Geometry check sheet. Reference: drawing and pictorial views, mm from the part's lowest x, y, z. A direction names the side the tool comes from. Coordinates: 2 decimals unless noted, no trailing zeros. Write each loop counter-clockwise with the first axis right and the second up, starting at its lowest first coordinate (ties: lowest second). Pieces come first, ordered by that corner, then holes. Notation, with made-up numbers: (-11.5, 88.25) -> (45.5, 88.25) arc R13 ccw to (45.5, 97.25) -> close; hole circle Ø7 at (78, -13.75). An arc over 180 degrees is marked (long way). Use a Markdown table: item, result.
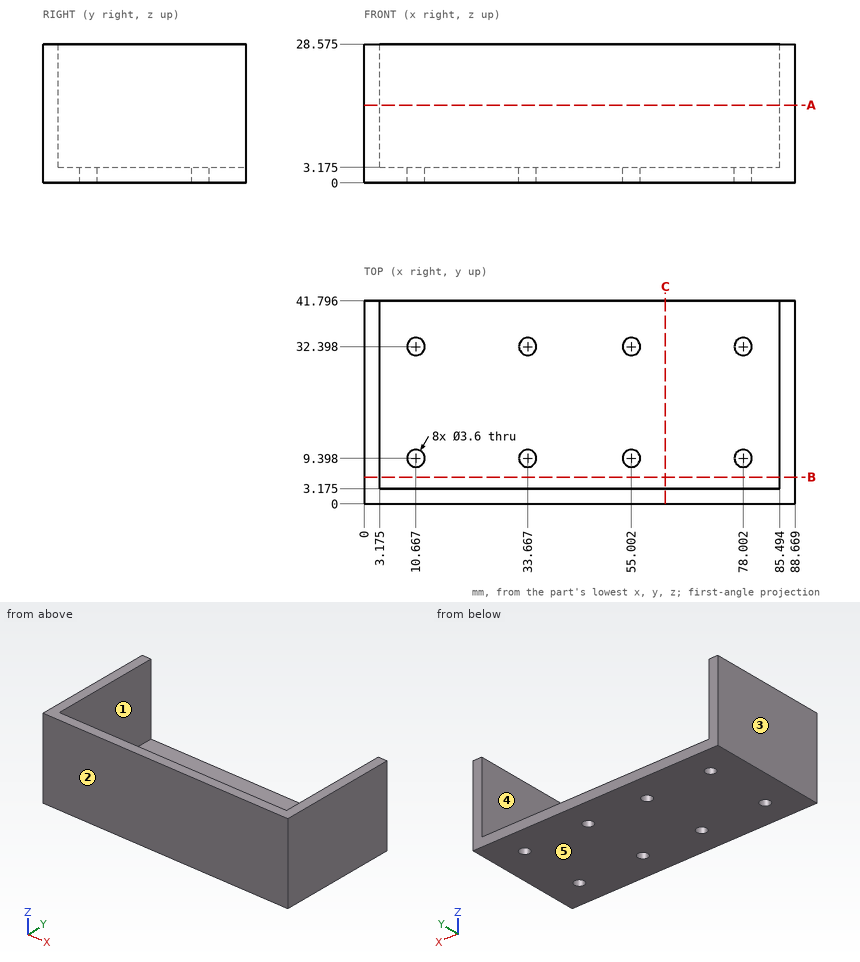
Item 1: Depth check by flat-ended pin: P1, Ø6, axis at x = 78, y = 32.4, coming from the +Z side (3 decimals); P2, Ø1.5, axis at x = 13.5, z = 23.5, coming from the +Y side (3 decimals). Enter the tip coordinate at first touch or a pass-through.
Answer block:
| item | result |
|---|---|
| P1 | stops at z = 3.175 |
| P2 | stops at y = 3.175 |
Item 2: Thickness scan on L1, parallel to X at y = 38.5, z = 15 (1 decimal); L2, parallel to X at y = 33, z = 2 (1 decimal); L3, parallel to Z at x = 42, y = 13 (1 decimal). Record the ranges inside material, lowest first. Write a range as [from, to].
Answer block:
| item | result |
|---|---|
| L1 | x = [0, 3.2], [85.5, 88.7] |
| L2 | x = [0, 9], [12.4, 32], [35.4, 53.3], [56.7, 76.3], [79.7, 88.7] |
| L3 | z = [0, 3.2] |
Item 3: Section check A-A on z = 16. Record the boundary of the cut face in (x, y) (1 decimal).
Answer block:
| item | result |
|---|---|
| outline | (0, 0) -> (88.7, 0) -> (88.7, 41.8) -> (85.5, 41.8) -> (85.5, 3.2) -> (3.2, 3.2) -> (3.2, 41.8) -> (0, 41.8) -> close |
Item 4: Mould release check, pull along X, two halves, no side actions. Record for the marked faces 1, 2 and 3: +X half, -X half, draft (parallel to the pull), parting line (faces both ways), or undercut.
Answer block:
| item | result |
|---|---|
| face 1 | undercut |
| face 2 | draft |
| face 3 | -X half |
Item 5: Section check C-C on x = 62. Record the boundary of the cut face in (y, z) (1 decimal).
Answer block:
| item | result |
|---|---|
| outline | (0, 0) -> (41.8, 0) -> (41.8, 3.2) -> (3.2, 3.2) -> (3.2, 28.6) -> (0, 28.6) -> close |
Item 6: Section check B-B on y = 5.5. Record the boundary of the cut face in (x, z) (1 decimal), then the cut area to 3 significant figures.
Answer block:
| item | result |
|---|---|
| outline | (0, 0) -> (88.7, 0) -> (88.7, 28.6) -> (85.5, 28.6) -> (85.5, 3.2) -> (3.2, 3.2) -> (3.2, 28.6) -> (0, 28.6) -> close |
| area | 443 mm^2 |
Item 7: Tool access check on the marked faces 4 and 5. Record the directions out of +Z, -Z, +X, -X, +Y, -Y that give a thin tool (end or side, any length) a straight path to the whole face; none if there is none.
Answer block:
| item | result |
|---|---|
| face 4 | +Z, +Y |
| face 5 | -Z, +X, -X, +Y, -Y |
